Source: CAD feature listing. Evaluate the final solid. Frame: model axes, mm. Face numbers are marked on the shaded views. Coordinates: 2 decimals unless noted, no trailing zeros. Loops run counter-clockwise (first coordinate to the right, second up) from the corner with the lowest first, then second, coordinate; pieces in that order, holes last. Notation, with made-up numbers: (37, 28.5) -> (46, 28.5) arc R36 cw to (46, 66.5) -> close; hole circle Ø4 at (-36.75, 50.25). An arc over 180 degrees is marked (long way). Answer as CSV lines item,"result".
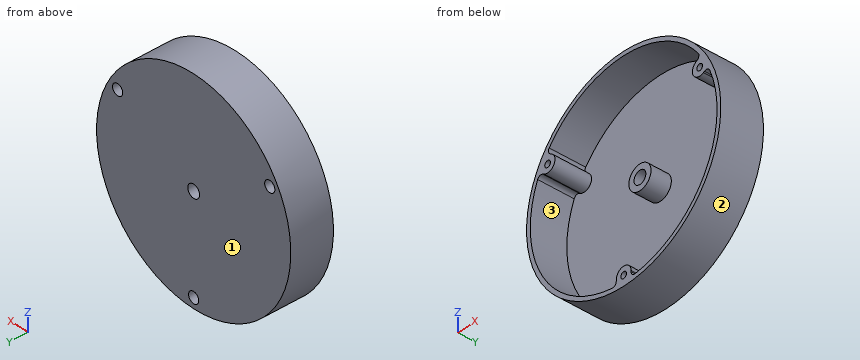
from build123d import *

# Parameters (mm, degrees)
ESQUISSE1_R             = 52.5
BOSS_EXTRU_1_DEPTH      = 18
ESQUISSE2_R             = 52.5
BOSS_EXTRU_2_DEPTH      = 3
ENL_V_START             = -3
ESQUISSE3_R             = 2.75
ENL_V_MAT_EXTRU_2_DEPTH = 75.158926898
ESQUISSE4_R             = 1.55
ENL_V_MAT_EXTRU_3_DEPTH = 78.158926898
ESQUISSE6_R             = 6
BOSS_EXTRU_3_DEPTH      = 10
ESQUISSE7_R             = 3.2
ENL_V_MAT_EXTRU_5_DEPTH = 78.158926898


with BuildPart() as part:
    # Esquisse1 → Boss.-Extru.1 (new body)
    with BuildSketch(Plane(origin=(0, 0, 0), x_dir=(1, 0, 0), z_dir=(0, 1, 0))):
        with Locations(Location((0, 0, 0), (0, 0, 270))):
            Circle(ESQUISSE1_R)
        with BuildLine():
            ThreePointArc((-4, 47.5), (0, 43.5), (4, 47.5))
            Line((4, 47.5), (4, 48.127435003))
            ThreePointArc((4, 48.127435003), (4.676150568, 49.626575651), (6.24742268, 50.112071498))
            ThreePointArc((6.24742268, 50.112071498), (43.734282891, 25.25), (46.522038294, -19.645609))
            ThreePointArc((46.522038294, -19.645609), (45.3159505, -20.763622642), (43.679581332, -20.599615887))
            Line((43.679581332, -20.599615887), (43.13620668, -20.285898385))
            ThreePointArc((43.13620668, -20.285898385), (37.672105065, -21.75), (39.13620668, -27.214101615))
            Line((39.13620668, -27.214101615), (39.679581332, -27.527819117))
            ThreePointArc((39.679581332, -27.527819117), (40.639799932, -28.862953009), (40.274615614, -30.466462499))
            ThreePointArc((40.274615614, -30.466462499), (0, -50.5), (-40.274615614, -30.466462499))
            ThreePointArc((-40.274615614, -30.466462499), (-40.639799932, -28.862953009), (-39.679581332, -27.527819117))
            Line((-39.679581332, -27.527819117), (-39.13620668, -27.214101615))
            ThreePointArc((-39.13620668, -27.214101615), (-37.672105065, -21.75), (-43.13620668, -20.285898385))
            Line((-43.13620668, -20.285898385), (-43.679581332, -20.599615887))
            ThreePointArc((-43.679581332, -20.599615887), (-45.3159505, -20.763622642), (-46.522038294, -19.645609))
            ThreePointArc((-46.522038294, -19.645609), (-43.734282891, 25.25), (-6.24742268, 50.112071498))
            ThreePointArc((-6.24742268, 50.112071498), (-4.676150568, 49.626575651), (-4, 48.127435003))
            Line((-4, 48.127435003), (-4, 47.5))
        make_face(mode=Mode.SUBTRACT)
    extrude(amount=BOSS_EXTRU_1_DEPTH)

    # Esquisse2 → Boss.-Extru.2 (add)
    with BuildSketch(Plane(origin=(0, 18, 0), x_dir=(1, 0, 0), z_dir=(0, 1, 0))):
        with Locations(Location((0, 0, 0), (0, 0, 270))):
            Circle(ESQUISSE2_R)
    extrude(amount=BOSS_EXTRU_2_DEPTH)

    # Esquisse3 → Enlèv. mat.-Extru.2 (cut, through all)
    with BuildSketch(Plane.XZ.offset(ENL_V_START)):
        with Locations(Location((0, -47.5, 0), (0, 0, 270))):
            Circle(ESQUISSE3_R)
        with Locations(Location((-41.13620668, 23.75, 0), (0, 0, 270))):
            Circle(ESQUISSE3_R)
        with Locations(Location((41.13620668, 23.75, 0), (0, 0, 270))):
            Circle(ESQUISSE3_R)
    extrude(amount=-ENL_V_MAT_EXTRU_2_DEPTH, mode=Mode.SUBTRACT)

    # Esquisse4 → Enlèv. mat.-Extru.3 (cut, through all)
    with BuildSketch(Plane.XZ):
        with Locations(Location((0, -47.5, 0), (0, 0, 270))):
            Circle(ESQUISSE4_R)
        with Locations(Location((-41.13620668, 23.75, 0), (0, 0, 270))):
            Circle(ESQUISSE4_R)
        with Locations(Location((41.13620668, 23.75, 0), (0, 0, 270))):
            Circle(ESQUISSE4_R)
    extrude(amount=-ENL_V_MAT_EXTRU_3_DEPTH, mode=Mode.SUBTRACT)

    # Esquisse6 → Boss.-Extru.3 (add)
    with BuildSketch(Plane.XZ.offset(-18)):
        with Locations(Location((0, 0, 0), (0, 0, 90))):
            Circle(ESQUISSE6_R)
    extrude(amount=BOSS_EXTRU_3_DEPTH)

    # Esquisse7 → Enlèv. mat.-Extru.5 (cut, through all)
    with BuildSketch(Plane(origin=(0, 21, 0), x_dir=(1, 0, 0), z_dir=(0, 1, 0))):
        with Locations(Location((0, 0, 0), (0, 0, 270))):
            Circle(ESQUISSE7_R)
    extrude(amount=-ENL_V_MAT_EXTRU_5_DEPTH, mode=Mode.SUBTRACT)


solid = part.part
(1) Cut plane C-C (x = 0). Return the cut outline in (y, z), then the cut area to 4 significant figures.
Computed values:
outline,"(0, -52.5) -> (21, -52.5) -> (21, -50.25) -> (3, -50.25) -> (3, -49.05) -> (0, -49.05) -> close; (0, -45.95) -> (3, -45.95) -> (3, -44.75) -> (21, -44.75) -> (21, -3.2) -> (8, -3.2) -> (8, -6) -> (18, -6) -> (18, -43.5) -> (0, -43.5) -> close; (0, 50.5) -> (18, 50.5) -> (18, 6) -> (8, 6) -> (8, 3.2) -> (21, 3.2) -> (21, 52.5) -> (0, 52.5) -> close"
area,"441.5 mm^2"
(2) Draft query along Z for the marked faces 1, 2 and 3. Return one class per face: released by +Z, released by -Z, zero draft, split by the parting line, or undercut.
Computed values:
face 1,"zero draft"
face 2,"split by the parting line"
face 3,"undercut"
(3) Cut plane D-D (z = 23.75). Return the cut outline in (x, y).
Computed values:
outline,"(-46.82, 0) -> (-42.69, 0) -> (-42.69, 3) -> (-43.89, 3) -> (-43.89, 21) -> (-46.82, 21) -> close; (-39.59, 0) -> (-37.14, 0) -> (-37.14, 18) -> (37.14, 18) -> (37.14, 0) -> (39.59, 0) -> (39.59, 3) -> (38.39, 3) -> (38.39, 21) -> (-38.39, 21) -> (-38.39, 3) -> (-39.59, 3) -> close; (42.69, 0) -> (46.82, 0) -> (46.82, 21) -> (43.89, 21) -> (43.89, 3) -> (42.69, 3) -> close"
(4) Cut plane A-A (y = 12). Return the cut outline in (x, z), then the cut area to 3 significant figures.
Computed values:
outline,"circle Ø105 at (0, 0); circle Ø12 at (0, 0); hole (-46.52, 19.65) arc R50.5 ccw to (-6.25, -50.11) arc R2 ccw to (-4, -48.13) -> (-4, -47.5) arc R4 cw to (4, -47.5) -> (4, -48.13) arc R2 ccw to (6.25, -50.11) arc R50.5 ccw to (46.52, 19.65) arc R2 ccw to (43.68, 20.6) -> (43.14, 20.29) arc R4 cw to (39.14, 27.21) -> (39.68, 27.53) arc R2 ccw to (40.27, 30.47) arc R50.5 ccw to (-40.27, 30.47) arc R2 ccw to (-39.68, 27.53) -> (-39.14, 27.21) arc R4 cw to (-43.14, 20.29) -> (-43.68, 20.6) arc R2 ccw to start; hole circle Ø5.5 at (-41.14, 23.75); hole circle Ø6.4 at (0, 0); hole circle Ø5.5 at (0, -47.5); hole circle Ø5.5 at (41.14, 23.75)"
area,"810 mm^2"
(5) Material intervals for L1, parallel to X at y = 1.2, z = 23.75; L2, parallel to Y at x = 31, z = 23; L3, parallel to Z at x = 39.5, y = 16.5, sorted ascending. Write a range as [from, to].
Computed values:
L1,"[-46.82, -42.69], [-39.59, -37.14], [37.14, 39.59], [42.69, 46.82]"
L2,"[18, 21]"
L3,"[-34.58, -31.46], [20.1, 21.54], [25.96, 27.42], [31.46, 34.58]"
(6) Pin query (flat end, axial travel): pin 1 Ø8 at (y, z) = (9.5, 23) entering from -X; pin 2 Ø1.6 at (x, z) = (0.5, -47.5) entering from +Y; pin 3 Ø1.6 at (x, z) = (-40, 25) entering from +Y; pin 4 Ø2 at (x, z) = (26.5, 15) entering from -Y. Return the tip coordinate at first contact, or that it passes through.
Computed values:
pin 1,"x = -48.94"
pin 2,"through"
pin 3,"y = 3"
pin 4,"y = 18"
(7) Cut plane B-B (z = 0). Return the cut outline in (x, y), then the cut area to 3 significant figures.
Computed values:
outline,"(-52.5, 0) -> (-50.5, 0) -> (-50.5, 18) -> (-6, 18) -> (-6, 8) -> (-3.2, 8) -> (-3.2, 21) -> (-52.5, 21) -> close; (3.2, 8) -> (6, 8) -> (6, 18) -> (50.5, 18) -> (50.5, 0) -> (52.5, 0) -> (52.5, 21) -> (3.2, 21) -> close"
area,"424 mm^2"
